Build history of the part. All positions in model axes, mm. A direction names the side the tool comes from. Round coordinates to 2 decimals unless told otherwise and drop trailing zeros. Write each loop counter-clockwise with the first axis right and the second up, starting at its lowest first coordinate (ties: lowest second). Pieces come first, ordered by that corner, then holes.
from build123d import *

# Parameters (mm, degrees)
F0_W      = 127
F0_H      = 25.4
F1_DEPTH  = 10.16
F2_R      = 3.5687
F3_DEPTH  = 3.048
F4_T      = -2.54
F5_R      = 4.7444277968
F5_R_2    = 3.6400744996
F6_DEPTH  = 5.588
F7_W      = 34.0172694892
F7_H      = 25.4
F8_DEPTH  = 25.4
F9_W      = 10.16
F9_H      = 25.4
F10_DEPTH = 1.3716


with BuildPart() as f1:
    # F0 (on Front) → F1 (new body)
    with BuildSketch(Plane.XZ):
        with Locations((10.5785235435, 35.8232918932)):
            Rectangle(F0_W, F0_H)
    extrude(amount=F1_DEPTH)

    # F2 (on face) → F3 (join)
    with BuildSketch(Plane.XZ.offset(10.16)):
        with Locations((-46.0632033646, 41.9265590608)):
            Circle(F2_R)
        with Locations((-46.0632033646, 29.322706577)):
            Circle(F2_R)
        with BuildLine():
            ThreePointArc((-31.0645033646, 41.9265590608), (-31.9468505317, 44.2758415358), (-34.1575782363, 45.4634221381))
            Line((-34.1575782363, 45.4634221381), (-34.0381698666, 38.4078157019))
            ThreePointArc((-34.0381698666, 38.4078157019), (-31.9074818331, 39.6230700066), (-31.0645033646, 41.9265590608))
        make_face()
        with BuildLine():
            ThreePointArc((-31.0645033646, 29.322706577), (-31.8767248088, 31.5892999815), (-33.9436726204, 32.8241587104))
            Line((-33.9436726204, 32.8241587104), (-33.8255849878, 25.8465920439))
            ThreePointArc((-33.8255849878, 25.8465920439), (-31.8387653718, 27.1030813847), (-31.0645033646, 29.322706577))
        make_face()
        with BuildLine():
            Line((-33.8255849878, 25.8465920439), (-33.9436726204, 32.8241587104))
            ThreePointArc((-33.9436726204, 32.8241587104), (-38.2013924038, 29.2623189066), (-33.8255849878, 25.8465920439))
        make_face()
        with BuildLine():
            Line((-34.0381698666, 38.4078157019), (-34.1575782363, 45.4634221381))
            ThreePointArc((-34.1575782363, 45.4634221381), (-38.2013924038, 41.8661713904), (-34.0381698666, 38.4078157019))
        make_face()
        with Locations((-23.2032033646, 41.9265590608)):
            Circle(F2_R)
        with Locations((-23.2032033646, 29.322706577)):
            Circle(F2_R)
        with Locations((-11.7732033646, 41.9265590608)):
            Circle(F2_R)
        with Locations((-11.7732033646, 29.322706577)):
            Circle(F2_R)
        with Locations((-0.3432033646, 41.9265590608)):
            Circle(F2_R)
        with Locations((-0.3432033646, 29.322706577)):
            Circle(F2_R)
        with Locations((11.0867966354, 41.9265590608)):
            Circle(F2_R)
        with Locations((11.0867966354, 29.322706577)):
            Circle(F2_R)
        with Locations((22.5167966354, 41.9265590608)):
            Circle(F2_R)
        with Locations((22.5167966354, 29.322706577)):
            Circle(F2_R)
        with Locations((33.9467966354, 41.9265590608)):
            Circle(F2_R)
        with Locations((33.9467966354, 29.322706577)):
            Circle(F2_R)
    extrude(amount=F3_DEPTH)

    # F4
    f4_openings = [f1.faces().sort_by_distance(p)[0] for p in [
        (10.578524, 0, 35.823292),
    ]]
    offset(amount=F4_T, openings=f4_openings, kind=Kind.INTERSECTION)

    # F5 (on face) → F6 (join)
    with BuildSketch(Plane(origin=(0, -7.62, 0), x_dir=(-1, 0, 0), z_dir=(0, 1, 0))):
        with Locations((37.8398224711, 35.6608107686)):
            Circle(F5_R)
        with Locations((37.8398224711, 35.6608107686)):
            Circle(F5_R_2, mode=Mode.SUBTRACT)
        with Locations((22.0918224711, 35.6608107686)):
            Circle(F5_R)
        with Locations((22.0918224711, 35.6608107686)):
            Circle(F5_R_2, mode=Mode.SUBTRACT)
        with Locations((6.3438224711, 35.6608107686)):
            Circle(F5_R)
        with Locations((6.3438224711, 35.6608107686)):
            Circle(F5_R_2, mode=Mode.SUBTRACT)
        with Locations((-9.4041775289, 35.6608107686)):
            Circle(F5_R)
        with Locations((-9.4041775289, 35.6608107686)):
            Circle(F5_R_2, mode=Mode.SUBTRACT)
        with Locations((-25.1521775289, 35.6608107686)):
            Circle(F5_R)
        with Locations((-25.1521775289, 35.6608107686)):
            Circle(F5_R_2, mode=Mode.SUBTRACT)
        with Locations((-40.9001775289, 35.6608107686)):
            Circle(F5_R)
        with Locations((-40.9001775289, 35.6608107686)):
            Circle(F5_R_2, mode=Mode.SUBTRACT)
        with Locations((-56.6481775289, 35.6608107686)):
            Circle(F5_R)
        with Locations((-56.6481775289, 35.6608107686)):
            Circle(F5_R_2, mode=Mode.SUBTRACT)
    extrude(amount=F6_DEPTH)

    # F7 (on face) → F8 (cut)
    with BuildSketch(Plane.XZ.offset(10.16)):
        with Locations((57.0698887989, 35.8232918932)):
            Rectangle(F7_W, F7_H)
    extrude(amount=-F8_DEPTH, mode=Mode.SUBTRACT)

    # F9 (on face) → F10 (join)
    with BuildSketch(Plane.YZ.offset(40.0612540543)):
        with Locations((-5.08, 35.8232918932)):
            Rectangle(F9_W, F9_H)
    extrude(amount=F10_DEPTH)


solid = f1.part
1) Mould opens along Z. For faces 1 (the cylindrical face through (9.88, -4.87, 39.27)), 2 (the flat face through (-35, -13.208, 42)) say: released by +Z, released by -Z, zero draft, split by the parting line, or undercut.
Results:
face 1: undercut
face 2: zero draft
2) Which spindle directions (+Z, -Z, +X, -X, +Y, -Y) get a long thin tool onto all of the face, cutting with end or side? Do faces 3 (the cylindrical face through (-46.53, -11.66, 32.86)), 4 (the cylindrical face through (-34.343, -4.865, 38.867)), 5 (the flat face through (34, -13.208, 42)). Say none if no direction does.
Results:
face 3: -Y
face 4: +Y
face 5: +Z, -Z, +X, -X, -Y
3) Slice it at C-C (x = -37). Write the cut outline in (y, z), plus the area to 3 significant figures.
Results:
outline: (-13.21, 26.65) - (-10.16, 26.65) - (-10.16, 23.12) - (0, 23.12) - (0, 25.66) - (-7.62, 25.66) - (-7.62, 30.99) - (-2.03, 30.99) - (-2.03, 32.12) - (-7.62, 32.12) - (-7.62, 39.2) - (-2.03, 39.2) - (-2.03, 40.33) - (-7.62, 40.33) - (-7.62, 45.98) - (0, 45.98) - (0, 48.52) - (-10.16, 48.52) - (-10.16, 44.6) - (-13.21, 44.6) - (-13.21, 39.26) - (-10.16, 39.26) - (-10.16, 31.99) - (-13.21, 31.99) - close
area: 148 mm2
4) Slice it at B-B (x = -7). Write the cut outline in (y, z), plus the area to 3 significant figures.
Results:
outline: (-10.16, 23.12) - (0, 23.12) - (0, 25.66) - (-7.62, 25.66) - (-7.62, 30.96) - (-2.03, 30.96) - (-2.03, 32.08) - (-7.62, 32.08) - (-7.62, 39.24) - (-2.03, 39.24) - (-2.03, 40.36) - (-7.62, 40.36) - (-7.62, 45.98) - (0, 45.98) - (0, 48.52) - (-10.16, 48.52) - close
area: 116 mm2
5) Wall check: L1, parallel to Z at x = -22, y = -3; L2, parallel to X at y = -1, z = 34; L3, parallel to Z at x = -34.5, y = -6. Give the ranges that are in metal, low to high.
Results:
L1: z = 23.12 to 25.66, 30.92 to 32.02, 39.3 to 40.4, 45.98 to 48.52
L2: x = -52.92 to -50.38, 40.06 to 41.43
L3: z = 23.12 to 25.66, 32.29 to 34.21, 37.11 to 39.03, 45.98 to 48.52
6) Slice it at A-A (y = -8.5). Count the separate pieces of the cut face and the enclosed holes in it, plus the area to 3 significant figures.
Results:
separate pieces: 1
enclosed holes: 16
area: 2,340 mm2
7) Pin check, flat tips, straight feed: pin 1 Ø2 at (x, z) = (-5.5, 35.5) entering from +Y; pin 2 Ø1 at (x, z) = (-23.5, 29.5) entering from +Y; pin 3 Ø6.5 at (x, z) = (-37.84, 35.66) entering from -Y. Stop position of each tip, or through.
Results:
pin 1: stops at y = -7.62
pin 2: stops at y = -10.67
pin 3: stops at y = -10.16
